Source: CAD feature listing. Evaluate the final solid. Frame: model axes, mm. Face numbers are marked on the shaded views. A direction names the side the tool comes from. Round coordinates to 2 decimals unless told otherwise and drop trailing zeros. Loops run counter-clockwise (first coordinate to the right, second up) from the corner with the lowest first, then second, coordinate; pieces in that order, holes last.
(1) Section C-C, the plane y = -5. Return the cut outline in (x, z), plus the area to 3 significant figures.
(2) Section B-B, the plane x = -7. Return the cut outline in (y, z), plus the area to 3 significant figures.
(3) First-contact query: pin 1 Ø1.8 at (y, z) = (5, 4) entering from -X; pin 2 Ø3 at (x, z) = (-14.5, 2.5) entering from -Y; pin 3 Ø1.5 at (y, z) = (-9.5, 1) entering from -X. Flat tips, straight axial feed; report the tip coordinate or a pass-through.
(4) Material intervals for probe 1 along Y at (x, z) = (-0.5, 4.6); probe 2 along Y at (x, z) = (1.5, 4.1); probe 3 along X at (y, z) = (5.5, 4.75), sorted ascending.
(5) Set-up query: the marked faces 1, 2 and 3. Return all of +Z, -Z, +X, -X, +Y, -Y with unobstructed straight access to the full face (end or side cutting, diameter ignored); none if empty.
(6) Mould query, pull axis X, two halves, no side actions, for the marked faces 4, 5 and 6. Classes: pulls with the +X half, pulls with the -X half, needs draft (parallel to the pull), parting line crosses it, or undercut.
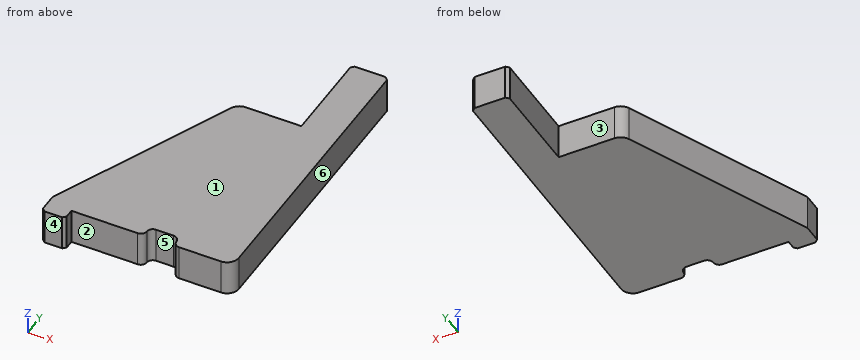
Autodesk Inventor part; units mm, degrees
ref_plane "YZ Plane" through (0, 0, 0) normal (1, 0, 0) x (0, 1, 0)
ref_plane "XZ Plane" through (0, 0, 0) normal (0, 1, 0) x (-1, 0, 0)
ref_plane "XY Plane" through (0, 0, 0) normal (0, 0, 1) x (1, 0, 0)
ref_plane "Work Plane1" through (0, 0, 0) normal (0, 0, 1) x (1, 0, 0)
sketch "Sketch1" plane through (0, 0, 0) normal (0, 0, 1) x (1, 0, 0)
  line L0 (0, 0) -> (6.2, 0)
  line L1 (0, 0) -> (0, -6)
  line L2 (6.2, -6) -> (0, -6)
  line L3 (6.2, 0) -> (6.2, -6)
  line L4 (6.2, -14.15) -> (12.2, -14.15)
  line L5 (6.2, -6) -> (6.2, -14.15)
  line L6 (-8.8, -6) -> (6.2, -6)
  line L7 (-24.1812, -40.5) -> (-8.8, -6)
  line L8 (6.2, -40.5) -> (-24.1812, -40.5)
  line L9 (6.2, -34.15) -> (6.2, -40.5)
  line L10 (12.2, -34.15) -> (6.2, -34.15)
  line L11 (12.2, -14.15) -> (12.2, -34.15)
  line L12 (-26.0293, -42.3) -> (-19.9707, -42.3)
  line L13 (6.2, -14.15) -> (12.2, -14.15)
  line L14 (6.2, -6) -> (6.2, -14.15)
  line L15 (-8.8, -6) -> (6.2, -6)
  line L16 (-24.1812, -40.5) -> (-8.8, -6)
  line L17 (6.2, -40.5) -> (-24.1812, -40.5)
  line L18 (6.2, -34.15) -> (6.2, -40.5)
  line L19 (12.2, -34.15) -> (6.2, -34.15)
  line L20 (12.2, -14.15) -> (12.2, -34.15)
  line L21 (6.2, -39.5) -> (-20.9707, -39.5)
  line L22 (6.2, 10) -> (0, 10)
  line L23 (0, 10) -> (0, -6)
  line L24 (-20.9707, -39.5) -> (-20.9707, -41.5)
  line L25 (-20.9707, -41.5) -> (-24.9707, -41.5)
  line L26 (0, -6) -> (-8.8, -6)
  line L27 (-24.9707, -41.5) -> (-24.9707, -38)
  line L28 (-24.9707, -38) -> (-10.704, -6)
  line L29 (-10.704, -6) -> (-8.8, -6)
  line L30 (6.2, -39.5) -> (6.2, 10)
  dimension "d1" = 1
  dimension "d3" = 4
  dimension "d4" = 1
  dimension "d5" = 2
  dimension "d6" = 3.5
  dimension "d7" = 10
extrude "Plate1" add sketch "Sketch1" along normal blind 6 contours L23 L22 L30 L0 | L0 L3 L2 L1 | L2 L5 L30 L9 L21 L24 L8 L7 L6 | L7 L8 L24 L25 L27 L28 L29
sketch "Sketch2" plane through (0, 0, 6) normal (0, 0, 1) x (1, 0, 0)
  line L0 (6.2, 10) -> (6.2, -39.5)
  line L1 (0, 10) -> (6.2, 10)
  line L2 (0, -6) -> (0, 10)
  line L3 (-10.704, -6) -> (0, -6)
  line L4 (-24.9707, -38) -> (-10.704, -6)
  line L5 (-24.9707, -41.5) -> (-24.9707, -38)
  line L6 (-20.9707, -41.5) -> (-24.9707, -41.5)
  line L7 (-20.9707, -39.5) -> (-20.9707, -41.5)
  line L8 (6.2, -39.5) -> (-20.9707, -39.5)
  line L9 (-8.8, -39.5) -> (-3.8, -39.5)
  line L10 (-3.8, -39.5) -> (-3.8, -37.5)
  line L11 (-3.8, -37.5) -> (-8.8, -37.5)
  line L12 (-8.8, -37.5) -> (-8.8, -39.5)
  point P0 (0, 0)
  dimension "d9" = 5
  dimension "d10" = 2
  dimension "d11" = 10
extrude "Cut1" cut sketch "Sketch2" against normal blind 6 contours L8 L12 L11 L10
fillet "Corner Round1" radius 1 4 edges at (-8.8, -39.5, 3) (-8.8, -37.5, 3) (-3.8, -37.5, 3) (-3.8, -39.5, 3)
chamfer "Corner Chamfer1" distance 0.5 angle 45 2 edges at (-24.9707, -41.5, 3) (-20.9707, -41.5, 3)
chamfer "Corner Chamfer2" distance 0.5 angle 45 2 edges at (0, 10, 3) (6.2, 10, 3)
fillet "Corner Round2" radius 2 2 edges at (-10.704, -6, 3) (6.2, -39.5, 3)
equation "\"d12\" = Thickness"
equation "\"d8\" = Thickness"
equation "\"BendRadius\" = Thickness"
equation "\"BendReliefWidth\" = Thickness"
equation "\"BendReliefDepth\" = 0.5 * Thickness"
equation "\"CornerReliefSize\" = 4 * Thickness"
equation "\"MinimumRemnant\" = 2 * Thickness"
equation "\"TransitionRadius\" = BendRadius"
equation "\"JacobiRadiusSize\" = BendRadius"
equation "\"GapSize\" = Thickness"
properties part number "knop nuc" material "Wood (Birch)"
Output values:
1. outline: (0, 0) - (6.2, 0) - (6.2, 6) - (0, 6) - close
1. area: 37.2 mm2
2. outline: (-37.5, 0) - (-6, 0) - (-6, 6) - (-37.5, 6) - close
2. area: 189 mm2
3. pin 1: stops at x = 0
3. pin 2: stops at y = -39.5
3. pin 3: stops at x = -12.6
4. probe 1: y = -39.5 to -6
4. probe 2: y = -39.5 to 10
4. probe 3: x = 0 to 6.2
5. face 1: +Z, +X, -X, +Y, -Y
5. face 2: +Z, -Z, +X, -Y
5. face 3: +Z, -Z, -X, +Y
6. face 4: needs draft
6. face 5: undercut
6. face 6: pulls with the +X half
